Build history of the part. All positions in model axes, mm. Round coordinates to 2 decimals unless told otherwise and drop trailing zeros. Loops run counter-clockwise (first coordinate to the right, second up) from the corner with the lowest first, then second, coordinate; pieces in that order, holes last.
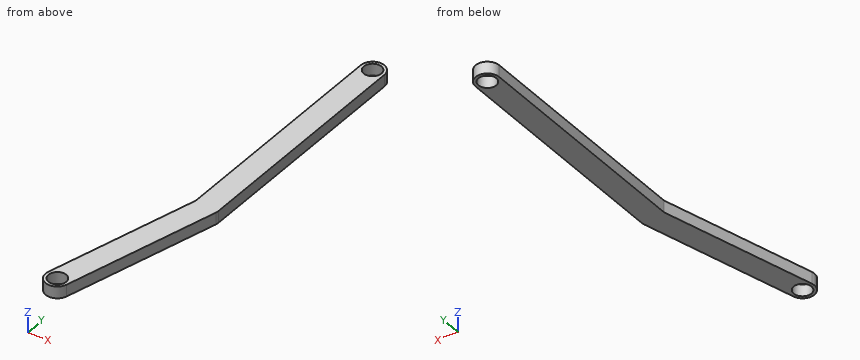
from build123d import *

# Parameters (mm, degrees)
SKETCH1_R           = 0.75
BOSS_EXTRUDE1_DEPTH = 1


with BuildPart() as part:
    # Sketch1 → Boss-Extrude1 (new body)
    with BuildSketch(Plane.XY):
        with BuildLine():
            Line((-2.517413675, -33.258819045), (0.965925826, -20.258819045))
            ThreePointArc((0.965925826, -20.258819045), (-0.130526192, -20.991444861), (-1, -20))
            Line((-1, -20), (-1, -19.868347502))
            Line((-1, -19.868347502), (-4.449265328, -32.741180955))
            ThreePointArc((-4.449265328, -32.741180955), (-3.742158547, -33.965925826), (-2.517413675, -33.258819045))
        make_face()
        with Locations((-3.483339502, -33)):
            Circle(SKETCH1_R, mode=Mode.SUBTRACT)
        with BuildLine():
            ThreePointArc((0.965925826, -20.258819045), (0.991444861, -20.130526192), (1, -20))
            ThreePointArc((1, -20), (0.130526192, -19.008555139), (-0.965925826, -19.741180955))
            Line((-0.965925826, -19.741180955), (-1, -19.868347502))
            Line((-1, -19.868347502), (-1, -20))
            ThreePointArc((-1, -20), (-0.130526192, -20.991444861), (0.965925826, -20.258819045))
        make_face()
        with BuildLine():
            Line((1, -20), (1, 0))
            ThreePointArc((1, 0), (0, 1), (-1, 0))
            Line((-1, 0), (-1, -19.868347502))
            Line((-1, -19.868347502), (-0.965925826, -19.741180955))
            ThreePointArc((-0.965925826, -19.741180955), (0.130526192, -19.008555139), (1, -20))
        make_face()
        Circle(SKETCH1_R, mode=Mode.SUBTRACT)
    extrude(amount=BOSS_EXTRUDE1_DEPTH)


solid = part.part
(1) Slice it at B-B on x = 0. List the corners of the cut face in (y, z).
Responses:
outline: (-23.86, 0) - (-0.75, 0) - (-0.75, 1) - (-23.86, 1) - close; (0.75, 0) - (1, 0) - (1, 1) - (0.75, 1) - close
(2) Slice it at A-A on z = 0.8. List the corners of the cut face in (x, y), plus the area to 3 significant figures.
Responses:
outline: (-4.45, -32.74) arc R1 ccw to (-2.52, -33.26) - (0.97, -20.26) arc R1 ccw to (1, -20) - (1, 0) arc R1 ccw to (-1, 0) - (-1, -19.87) - close; hole circle Ø1.5 at (-3.48, -33); hole circle Ø1.5 at (0, 0)
area: 66.5 mm2
(3) Slice it at C-C on y = -2. List the corners of the cut face in (x, z), plus the area to 3 significant figures.
Responses:
outline: (-1, 0) - (1, 0) - (1, 1) - (-1, 1) - close
area: 2.00 mm2
(4) Pin check, flat tip, straight feed: P1, Ø0.5, axis at y = -10.5, z = 0.5, coming from the -X side. Stop position of the tip, or through.
Responses:
P1: stops at x = -1
(5) Probe line 1 (X direction, y = -16, z = 0.95); line 2 (X direction, y = -24, z = 0.7). List the from-to ranges inside material, lowest first.
Responses:
line 1: x = -1 to 1
line 2: x = -2.11 to -0.04
(6) Slice it at D-D on x = -1.9. List the corners of the cut face in (y, z), plus the area to 3 significant figures.
Responses:
outline: (-30.95, 0) - (-23.23, 0) - (-23.23, 1) - (-30.95, 1) - close
area: 7.73 mm2
